```python
from build123d import *

# Parameters (mm, degrees)
SKETCH1_R           = 1.125
BOSS_EXTRUDE1_DEPTH = 5


with BuildPart() as part:
    # Sketch1 → Boss-Extrude1 (new body)
    with BuildSketch(Plane(origin=(0, 0, 0), x_dir=(1, 0, 0), z_dir=(0, 1, 0))):
        with BuildLine():
            ThreePointArc((-3.745309567, 0.1875), (0, -3.75), (3.745309567, 0.1875))
            Line((3.745309567, 0.1875), (1.997498436, 35.1))
            ThreePointArc((1.997498436, 35.1), (0, 37), (-1.997498436, 35.1))
            Line((-1.997498436, 35.1), (-3.745309567, 0.1875))
        make_face()
        with Locations(Location((0, 0, 0), (0, 0, 270))):
            Circle(SKETCH1_R, mode=Mode.SUBTRACT)
        with Locations(Location((0, 35, 0), (0, 0, 270))):
            Circle(SKETCH1_R, mode=Mode.SUBTRACT)
    extrude(amount=BOSS_EXTRUDE1_DEPTH)


solid = part.part
```
Can you work these out from the model? Positions are in its coordinate system, mm. Coordinates: 2 decimals unless noted, no trailing zeros. Loops run counter-clockwise (first coordinate to the right, second up) from the corner with the lowest first, then second, coordinate; pieces in that order, holes last. Notation, with made-up numbers: (51, -37.75) - (57, -37.75) arc R17 cw to (57, -12.75) - close; hole circle Ø11 at (-0.5, 7.5). An arc over 180 degrees is marked (long way). Use a Markdown table: item, result.
Item 1: If I drill on probe 1 along X at (y, z) = (1.6, 0) (3 decimals); probe 2 along X at (y, z) = (4.65, 1); probe 3 along X at (y, z) = (1.4, -23.5), over which ranges is the centre line in solid material (lowest first)? Write a range as from..to.
Numbers:
| item | result |
|---|---|
| probe 1 | x = -3.75..-1.125, 1.125..3.75 |
| probe 2 | x = -3.61..-0.52, 0.52..3.61 |
| probe 3 | x = -2.58..2.58 |
Item 2: I want a section at A-A on x = 0. Please give me the cut outline in (y, z) (3 decimals).
Numbers:
| item | result |
|---|---|
| outline | (0, -37) - (5, -37) - (5, -36.125) - (0, -36.125) - close; (0, -33.875) - (5, -33.875) - (5, -1.125) - (0, -1.125) - close; (0, 1.125) - (5, 1.125) - (5, 3.75) - (0, 3.75) - close |
Item 3: We'd pull the mould along X, two halves only. Please class faces 1 (the face through (-0.43, 2.46, -33.96)), 2 (the face through (0, 5, -12)), 3 (the face through (0, 2, -37)): released by +X, released by -X, zero draft, split by the parting line, or undercut.
Numbers:
| item | result |
|---|---|
| face 1 | undercut |
| face 2 | zero draft |
| face 3 | split by the parting line |
Item 4: Will this pin go through, and if not, where does the flat tip stop? pin 1 (3 mm diameter, centred on x = 1.5, y = 3, fed in from -Z).
Numbers:
| item | result |
|---|---|
| pin 1 | stops at z = -37 |
Item 5: I want a section at B-B on y = 1.15. Give the number of separate pieces and of enclosed holes in the cut face, and give its area (3 significant figures).
Numbers:
| item | result |
|---|---|
| separate pieces | 1 |
| enclosed holes | 2 |
| area | 222 mm2 |
Item 6: I want a section at D-D on x = -1.5. Please give me the cut outline in (y, z), and give its area (3 significant figures).
Numbers:
| item | result |
|---|---|
| outline | (0, -36.32) - (5, -36.32) - (5, 3.44) - (0, 3.44) - close |
| area | 199 mm2 |
Item 7: I want a section at C-C on z = -5. Please give me the cut outline in (x, y).
Numbers:
| item | result |
|---|---|
| outline | (-3.5, 0) - (3.5, 0) - (3.5, 5) - (-3.5, 5) - close |
